```python
from build123d import *

# Parameters (mm, degrees)
SKETCH_1_W           = 50
SKETCH_1_H           = 40
EXTRUDE_1_DEPTH      = 8
CHAMFER_1_SIZE       = 10
SKETCH_2_R           = 1.55
CUT_EXTRUDE_1_DEPTH  = 10
EXTRUDE_2_DEPTH      = 30
EXTRUDE_2_DEPTH_BACK = 15
SKETCH_3_R           = 12.5
SKETCH_4_R           = 1.7
CUT_EXTRUDE_2_DEPTH  = 15
CUT_EXTRUDE_START    = -20
CUT_EXTRUDE_3_DEPTH  = 20
SKETCH_7_R           = 16.5
CUT_EXTRUDE_8_DEPTH  = 33
CUT_EXTRUDE_9_DEPTH  = 20
CHAMFER_3_SIZE       = 2
CUT_EXTRUDE_START_2  = 20
SKETCH_10_OUTSIDE_W  = 45.574
SKETCH_10_OUTSIDE_H  = 60.574
SKETCH_10_OUTSIDE_R  = 12.466047995
CUT_EXTRUDE_10_DEPTH = 10
CHAMFER_4_SIZE       = 10
SKETCH_14_W          = 12
SKETCH_14_H          = 23
CUT_EXTRUDE_11_DEPTH = 3
CUT_EXTRUDE_12_DEPTH = 4.2
SKETCH_16_R          = 1.1
CUT_EXTRUDE_13_DEPTH = 5
SKETCH_17_R          = 3.372674955
EXTRUDE_3_DEPTH      = 4
SKETCH_18_R          = 1.1
CUT_EXTRUDE_14_DEPTH = 4
SKETCH_20_R          = 4
CUT_EXTRUDE_15_DEPTH = 4
CUT_EXTRUDE_17_DEPTH = 10


# Read off the part's stored shape, not the designer's step: 切除-拉伸3
with BuildPart() as part:
    # 草图1 → 凸台-拉伸1 (new body)
    with BuildSketch(Plane.XY):
        Rectangle(SKETCH_1_W, SKETCH_1_H)
    extrude(amount=EXTRUDE_1_DEPTH)

    # 倒角1
    chamfer_1_edges = [part.edges().sort_by_distance(p)[0] for p in [
        (-25, -20, 4),
        (-25, 20, 4),
    ]]
    chamfer(chamfer_1_edges, length=CHAMFER_1_SIZE)

    # 草图2 → 切除-拉伸1 (cut)
    with BuildSketch(Plane.XY.offset(8)):
        with Locations((-2, -10)):
            Circle(SKETCH_2_R)
        with Locations((-2, 10)):
            Circle(SKETCH_2_R)
    extrude(amount=-CUT_EXTRUDE_1_DEPTH, mode=Mode.SUBTRACT)

    # 草图3 → 凸台-拉伸2 (add, two sides: drawn at the far end of the back side and taken through both)
    with BuildSketch(Plane(origin=(25, 0, 0), x_dir=(0, 0, -1), z_dir=(1, 0, 0)).offset(-EXTRUDE_2_DEPTH_BACK)):
        with Locations(Location((-4, 0, 0), (0, 0, 251.337075115))):
            Circle(SKETCH_3_R)
    extrude(amount=EXTRUDE_2_DEPTH + EXTRUDE_2_DEPTH_BACK)

    # 草图4 → 切除-拉伸2 (cut)
    with BuildSketch(Plane.XY.offset(8)):
        with Locations((-19.690178066, -4)):
            Circle(SKETCH_4_R)
        with Locations((-19.690178066, 4)):
            Circle(SKETCH_4_R)
    extrude(amount=-CUT_EXTRUDE_2_DEPTH, mode=Mode.SUBTRACT)

    # 切除-拉伸3 outline → 切除-拉伸3 (cut)
    with BuildSketch(Plane(origin=(55, 0, 0), x_dir=(0, 0, -1), z_dir=(1, 0, 0)).offset(CUT_EXTRUDE_START)):
        with BuildLine():
            Line((7.456439237, -5), (-15.456439237, -5))
            ThreePointArc((-15.456439237, -5), (-4, -12.5), (7.456439237, -5))
        make_face()
        with BuildLine():
            ThreePointArc((7.456439237, 5), (-4, 12.5), (-15.456439237, 5))
            Line((-15.456439237, 5), (7.456439237, 5))
        make_face()
    extrude(amount=CUT_EXTRUDE_3_DEPTH, mode=Mode.SUBTRACT)

    # 草图7 → 切除-拉伸8 (cut)
    with BuildSketch(Plane.XZ.offset(5)):
        with Locations((38.5, 4)):
            Circle(SKETCH_7_R)
    cut_extrude_8 = extrude(amount=CUT_EXTRUDE_8_DEPTH, mode=Mode.SUBTRACT)

    # 镜向1: 切除-拉伸8 across plane
    add(cut_extrude_8.mirror(Plane.ZX), mode=Mode.SUBTRACT)

    # 草图8 → 切除-拉伸9 (cut)
    with BuildSketch(Plane.XZ.offset(5)):
        with BuildLine():
            Line((40, 19.107397707), (75.764252489, 33.62580965))
            Line((75.764252489, 33.62580965), (78.826270749, -18.347337912))
            Line((78.826270749, -18.347337912), (40, -10.892602293))
            ThreePointArc((40, -10.892602293), (55, 4.107397707), (40, 19.107397707))
        make_face()
    extrude(amount=-CUT_EXTRUDE_9_DEPTH, mode=Mode.SUBTRACT)

    # 倒角3
    chamfer_3_edges = [part.edges().sort_by_distance(p)[0] for p in [
        (10, 0, 16.5),
        (10, 0, -8.5),
    ]]
    chamfer(chamfer_3_edges, length=CHAMFER_3_SIZE)

    # 草图10 outside → 切除-拉伸10 (cut)
    with BuildSketch(Plane(origin=(10, 0, 0), x_dir=(0, 0, -1), z_dir=(1, 0, 0)).offset(CUT_EXTRUDE_START_2)):
        with Locations((-4, 0)):
            Rectangle(SKETCH_10_OUTSIDE_W, SKETCH_10_OUTSIDE_H)
        with Locations((-4.107397707, 0)):
            Circle(SKETCH_10_OUTSIDE_R, mode=Mode.SUBTRACT)
    extrude(amount=-CUT_EXTRUDE_10_DEPTH, mode=Mode.SUBTRACT)

    # 倒角4
    # the kernel refuses this chamfer: 10 mm, written as the material it takes off along each edge
    with BuildSketch(Plane(origin=(20, -20, -25.71682988), x_dir=(-0.9996219169112968, -0.027495876610586317, 0), z_dir=(0, 0, 1))) as chamfer_4_piece_1_section:
        Polygon((CHAMFER_4_SIZE * 0.999621916911, -CHAMFER_4_SIZE * 0.0274958766106), (-CHAMFER_4_SIZE * 0.0274958766106, -CHAMFER_4_SIZE * 0.999621916911), (0, 0), align=None)
    chamfer_4_piece_1 = extrude(amount=59.433659759, mode=Mode.PRIVATE)
    chamfer_4_piece_1 = chamfer_4_piece_1 - Plane(origin=(16.670068992, 0, 4.107397707), x_dir=(0, 0, -1), z_dir=(1, 0, 0)) * Cylinder(12.466047995, 159, mode=Mode.PRIVATE)
    add(chamfer_4_piece_1, mode=Mode.SUBTRACT)
    with BuildSketch(Plane(origin=(20, 20, 33.71682988), x_dir=(-0.9996219169112968, 0.027495876610586317, 0), z_dir=(0, 0, -1))) as chamfer_4_piece_2_section:
        Polygon((CHAMFER_4_SIZE * 0.999621916911, -CHAMFER_4_SIZE * 0.0274958766106), (-CHAMFER_4_SIZE * 0.0274958766106, -CHAMFER_4_SIZE * 0.999621916911), (0, 0), align=None)
    chamfer_4_piece_2 = extrude(amount=59.433659759, mode=Mode.PRIVATE)
    chamfer_4_piece_2 = chamfer_4_piece_2 - Plane(origin=(16.670068992, 0, 4.107397707), x_dir=(0, 0, -1), z_dir=(1, 0, 0)) * Cylinder(12.466047995, 159, mode=Mode.PRIVATE)
    add(chamfer_4_piece_2, mode=Mode.SUBTRACT)

    # 草图14 → 切除-拉伸11 (cut)
    with BuildSketch(Plane(origin=(0, 0, 0), x_dir=(-1, 0, 0), z_dir=(0, 0, -1))):
        with Locations((2, 4.65)):
            Rectangle(SKETCH_14_W, SKETCH_14_H)
    extrude(amount=-CUT_EXTRUDE_11_DEPTH, mode=Mode.SUBTRACT)

    # 草图15 → 切除-拉伸12 (cut)
    with BuildSketch(Plane(origin=(0, 0, 3), x_dir=(-1, 0, 0), z_dir=(0, 0, -1))):
        with BuildLine():
            ThreePointArc((4.631967524, 4.49702381), (2, 16.1), (-0.631967524, 4.49702381))
            ThreePointArc((-0.631967524, 4.49702381), (2, 0.95), (4.631967524, 4.49702381))
        make_face()
    extrude(amount=-CUT_EXTRUDE_12_DEPTH, mode=Mode.SUBTRACT)

    # 草图16 → 切除-拉伸13 (cut)
    with BuildSketch(Plane(origin=(0, 0, 0), x_dir=(-1, 0, 0), z_dir=(0, 0, -1))):
        with Locations((2, 18.3)):
            Circle(SKETCH_16_R)
    extrude(amount=-CUT_EXTRUDE_13_DEPTH, mode=Mode.SUBTRACT)

    # 草图17 → 凸台-拉伸3 (add)
    with BuildSketch(Plane(origin=(0, 0, 0), x_dir=(-1, 0, 0), z_dir=(0, 0, -1))):
        with Locations((2, -10)):
            Circle(SKETCH_17_R)
    extrude(amount=-EXTRUDE_3_DEPTH)

    # 草图18 → 切除-拉伸14 (cut)
    with BuildSketch(Plane(origin=(0, 0, 0), x_dir=(-1, 0, 0), z_dir=(0, 0, -1))):
        with Locations((2, -9)):
            Circle(SKETCH_18_R)
    extrude(amount=-CUT_EXTRUDE_14_DEPTH, mode=Mode.SUBTRACT)

    # 草图20 → 切除-拉伸15 (cut)
    with BuildSketch(Plane(origin=(0, 0, 7.2), x_dir=(-1, 0, 0), z_dir=(0, 0, -1))):
        with Locations((2, 10)):
            Circle(SKETCH_20_R)
    extrude(amount=-CUT_EXTRUDE_15_DEPTH, mode=Mode.SUBTRACT)

    # 草图21 → 切除-拉伸17 (cut)
    with BuildSketch(Plane.XZ.offset(5)):
        with BuildLine():
            Line((42.683281573, 7.207397707), (37.316718427, 7.207397707))
            ThreePointArc((37.316718427, 7.207397707), (38.295807295, 0.378359329), (44.1, 4.107397707))
            ThreePointArc((44.1, 4.107397707), (43.729038378, 5.811590412), (42.683281573, 7.207397707))
        make_face()
    extrude(amount=-CUT_EXTRUDE_17_DEPTH, mode=Mode.SUBTRACT)


solid = part.part
```
Model file for the job. Use its own axes, mm. A direction names the side the tool comes from. Coordinates: 2 decimals unless noted, no trailing zeros. Loops run counter-clockwise (first coordinate to the right, second up) from the corner with the lowest first, then second, coordinate; pieces in that order, holes last. Notation, with made-up numbers: (-16.75, -17.75) - (27.25, -17.75) arc R10 cw to (27.25, -7.75) - close; hole circle Ø10 at (10, 52). An arc over 180 degrees is marked (long way). Answer as a JSON object with one key per item and string values. Group by question number.
(1) Two-plate mould, pull along Y, no slides. Class faces 6 (the face through (35, 5, 4)), 7 (the face through (10.125, -0.185, -6.623)), 8 (the face through (-2, 18, 5)): released by +Y, released by -Y, zero draft, split by the parting line, or undercut.
(2) Cut at D-D (y = 15). Give the cut face in (x, z), then the cut area to 3 significant figures.
(3) Cut at A-A (x = -2). Give the cut face in (y, z).
(4) Cut at C-C (y = -4). State how many separate pieces and enclosed holes the cut face has, then the cut area to 3 significant figures.
(5) Tool access for faces 1 (the face through (0.3, 15.9, 3)), 2 (the face through (-2, -11, 4)), 3 (the face through (26.4, 0.2, 16.5)), 4 (the face through (-3, -20, 4)), 5 (the face through (10, 1, 11)): list every direction of +Z, -Z, +X, -X, +Y, -Y with a clear straight run to the whole face (end or side of a thin tool).
(6) Probe line 1 along Y through (x, z) = (-2, 2.8); line 2 along Y through (x, z) = (-2, 3.1); line 3 along X through (y, z) = (10, 4.55). List the from-to ranges inside material, lowest first.
(7) Cut at B-B (x = 15.5). Give the cut face in (y, z), then the cut area to 3 significant figures.
(8) Flat gauge pins, fed straight in: pin 1 (4 mm diameter, centred on x = -2, y = -10, fed in from -Z); pin 2 (13 mm diameter, centred on x = 40, z = 4.11, fed in from +Y); pin 3 (1.5 mm diameter, centred on x = -2, y = 14, fed in from -Z); pin 4 (4 mm diameter, centred on x = -1, y = 10, fed in from -Z). Where does each tip first touch, or does it go through?
Geometry says:
{
 "1": {"face 6": "released by +Y", "face 7": "split by the parting line", "face 8": "undercut"},
 "2": {"outline": "(-20, 0) - (-8, 0) - (-8, 3) - (-5.49, 3) - (-5.49, 7.2) - (1.49, 7.2) - (1.49, 3) - (4, 3) - (4, 0) - (15, 0) - (15, 8) - (-20, 8) - close", "area": "215 mm^2"},
 "3": {"outline": "(-20, 0) - (-10.1, 0) - (-10.1, 4) - (-11.55, 4) - (-11.55, 8) - (-20, 8) - close; (-8.45, 4) - (-7.9, 4) - (-7.9, 0) - (-6.63, 0) - (-6.63, 3) - (0.95, 3) - (0.95, 7.2) - (6, 7.2) - (6, 8) - (-8.45, 8) - close; (14, 7.2) - (16.1, 7.2) - (16.1, 3) - (16.15, 3) - (16.15, 0) - (17.2, 0) - (17.2, 5) - (19.4, 5) - (19.4, 0) - (20, 0) - (20, 8) - (14, 8) - close"},
 "4": {"separate pieces": "2", "enclosed holes": "1", "area": "1,190 mm^2"},
 "5": {"face 1": "-Z", "face 2": "+Z", "face 3": "+Z, +X, -X", "face 4": "+Z, -Z, +X, -X, -Y", "face 5": "+Z, -X, +Y, -Y"},
 "6": {"line 1": "y = -20 to -10.1, -7.9 to -6.63, 16.15 to 17.2, 19.4 to 20", "line 2": "y = -20 to -10.1, -7.9 to 0.95, 16.1 to 17.2, 19.4 to 20", "line 3": "x = -25 to -8.1, 4.1 to 22.01"},
 "7": {"outline": "(-14.5, 0) - (-11.84, 0) arc R12.5 ccw to (11.84, 0) - (14.5, 0) - (14.5, 8) - (11.84, 8) arc R12.5 ccw to (-11.84, 8) - (-14.5, 8) - close", "area": "526 mm^2"},
 "8": {"pin 1": "stops at z = 0", "pin 2": "stops at y = 5", "pin 3": "stops at z = 7.2", "pin 4": "passes through"}
}
